Read the model definition and answer for the solid it produces. Units are mm, in the model's axes. A direction names the side the tool comes from. Give positions to 0.01 mm unless a question says otherwise; leave off trailing zeros. Order: outer loops, then holes, each group sorted by start corner. A loop starts at its lowest first (then second) coordinate and runs counter-clockwise, first axis right, second up. Notation, with made-up numbers: (83, 54) - (104, 54) arc R23 ccw to (104, 65) - close; hole circle Ø7 at (42.25, 24.5). An arc over 180 degrees is marked (long way). Return JSON: item names as keys, results as strings.
```python
from build123d import *

# Parameters (mm, degrees)
ESBO_O1_R                  = 23
ESBO_O1_R_2                = 13.905
RESSALTO_EXTRUS_O1_DEPTH   = 11
ESBO_O2_R                  = 23
RESSALTO_EXTRUS_O2_DEPTH   = 5
ESBO_O3_R                  = 2.5
CORTE_EXTRUS_O1_DEPTH      = 18
ESBO_O4_R                  = 4.5
CORTE_EXTRUS_O2_DEPTH      = 4
ESBO_O6_R                  = 24.343049023
CORTE_EXTRUS_O4_DEPTH      = 2
CHANFRO1_SIZE              = 1
CORTE_EXTRUS_O5_DEPTH      = 30
CORTE_EXTRUS_O5_DEPTH_BACK = 31
ESBO_O7_R                  = 1.25


with BuildPart() as part:
    # Esboço1 → Ressalto-extrusão1 (new body)
    with BuildSketch(Plane.XY):
        Circle(ESBO_O1_R)
        Circle(ESBO_O1_R_2, mode=Mode.SUBTRACT)
    extrude(amount=RESSALTO_EXTRUS_O1_DEPTH)

    # Esboço2 → Ressalto-extrusão2 (add)
    with BuildSketch(Plane.XY.offset(11)):
        Circle(ESBO_O2_R)
    extrude(amount=RESSALTO_EXTRUS_O2_DEPTH)

    # Esboço3 → Corte-extrusão1 (cut)
    with BuildSketch(Plane.XY.offset(16)):
        Circle(ESBO_O3_R)
    extrude(amount=-CORTE_EXTRUS_O1_DEPTH, mode=Mode.SUBTRACT)

    # Esboço4 → Corte-extrusão2 (cut)
    with BuildSketch(Plane(origin=(0, 0, 11), x_dir=(-1, 0, 0), z_dir=(0, 0, -1))):
        Circle(ESBO_O4_R)
    extrude(amount=-CORTE_EXTRUS_O2_DEPTH, mode=Mode.SUBTRACT)

    # Esboço6 → Corte-extrusão4 (cut)
    with BuildSketch(Plane(origin=(0, 0, 0), x_dir=(-1, 0, 0), z_dir=(0, 0, -1))):
        Circle(ESBO_O6_R)
    extrude(amount=-CORTE_EXTRUS_O4_DEPTH, mode=Mode.SUBTRACT)

    # Chanfro1
    chanfro1_edges = [part.edges().sort_by_distance(p)[0] for p in [
        (-23, 0, 2),
    ]]
    chamfer(chanfro1_edges, length=CHANFRO1_SIZE)

    # Esboço7 → Corte-extrusão5 (cut, two sides: drawn at the far end of the back side and taken through both)
    with BuildSketch(Plane(origin=(0, 0, 0), x_dir=(1, 0, 0), z_dir=(0, 1, 0)).offset(-CORTE_EXTRUS_O5_DEPTH_BACK)):
        with Locations(Location((0, -13.09796997, 0), (0, 0, 90))):
            Circle(ESBO_O7_R)
    extrude(amount=CORTE_EXTRUS_O5_DEPTH + CORTE_EXTRUS_O5_DEPTH_BACK, mode=Mode.SUBTRACT)


solid = part.part
```
Q1. Given pin 1 (4 mm diameter, centred on x = -5.5, z = 8, fed in from -Y); pin 2 (7 mm diameter, centred on x = -1.5, y = 0.5, fed in from -Z); pin 3 (5 mm diameter, centred on x = 18, z = 11, fed in from -Y), each flat-ended and moving along its own axis, determine where each tip first touches the part or whether it passes through.
Values:
{"pin 1": "stops at y = -22.73", "pin 2": "stops at z = 11", "pin 3": "stops at y = -16.99"}
Q2. A cutting plane is placed at B-B (y = 0). Write down the section's boundary in (x, z) (3 decimals).
Values:
{"outline": "(-23, 3) - (-22, 2) - (-13.905, 2) - (-13.905, 11) - (-4.5, 11) - (-4.5, 15) - (-2.5, 15) - (-2.5, 16) - (-23, 16) - close; (2.5, 15) - (4.5, 15) - (4.5, 11) - (13.905, 11) - (13.905, 2) - (22, 2) - (23, 3) - (23, 16) - (2.5, 16) - close"}
Q3. Determine the mould class of faces 3 (the flat face through (-14.4, 0.3, 2)), 4 (the cylindrical face through (-4.16, -1.72, 12.97)), 5 (the cylindrical face through (-2.994, 22.804, 9.409)) for opening direction X: released by +X, released by -X, zero draft, split by the parting line, or undercut.
Values:
{"face 3": "zero draft", "face 4": "undercut", "face 5": "split by the parting line"}
Q4. For faces 1 (the cylindrical face through (-0.375, 13.531, 11.906)), 2 (the flat face through (-3.3, 3.3, 11)), determine the directions among +Z, -Z, +X, -X, +Y, -Y from which every point of the face is accessible in a straight line to the end or side of a thin tool.
Values:
{"face 1": "+Y, -Y", "face 2": "-Z"}
Q5. Consider L1, parallel to Y at x = 0, z = 7 (3 decimals); L2, parallel to Y at x = 0, z = 15.75. Determine where each line is inside the solid, lowest interval first.
Values:
{"L1": "y = -23 to -13.905, 13.905 to 23", "L2": "y = -23 to -2.5, 2.5 to 23"}
Q6. A cutting plane is placed at A-A (x = 0). Write down the section's boundary in (y, z) (3 decimals), and give its area (3 significant figures).
Values:
{"outline": "(-23, 3) - (-22, 2) - (-13.905, 2) - (-13.905, 11) - (-4.5, 11) - (-4.5, 11.848) - (-23, 11.848) - close; (-23, 14.348) - (-4.5, 14.348) - (-4.5, 15) - (-2.5, 15) - (-2.5, 16) - (-23, 16) - close; (2.5, 15) - (4.5, 15) - (4.5, 14.348) - (23, 14.348) - (23, 16) - (2.5, 16) - close; (4.5, 11) - (13.905, 11) - (13.905, 2) - (22, 2) - (23, 3) - (23, 11.848) - (4.5, 11.848) - close", "area": "259 mm²"}
